Source: CAD feature listing. Evaluate the final solid. Frame: model axes, mm. A direction names the side the tool comes from. Coordinates: 2 decimals unless noted, no trailing zeros. Order: outer loops, then holes, each group sorted by start corner. A loop starts at its lowest first (then second) coordinate and runs counter-clockwise, first axis right, second up. Notation, with made-up numbers: (72, 80.5) -> (111, 80.5) arc R28 cw to (111, 117.5) -> close; hole circle Ø1 at (79.5, 60.25). An arc over 180 degrees is marked (long way). Put each result on its own line as item: value.
from build123d import *

# Parameters (mm, degrees)
SKETCH2_W           = 67
SKETCH2_H           = 85
SKETCH2_W_2         = 57
SKETCH2_H_2         = 75
BOSS_EXTRUDE1_DEPTH = 4
SKETCH2_3_W         = 67
SKETCH2_3_H         = 85
SKETCH2_3_W_2       = 57
SKETCH2_3_H_2       = 75
BOSS_EXTRUDE2_DEPTH = 114
SKETCH4_W           = 67
SKETCH4_H           = 85
SKETCH4_W_2         = 63
SKETCH4_H_2         = 81
BOSS_EXTRUDE3_DEPTH = 25
SKETCH6_R           = 8
CUT_EXTRUDE1_DEPTH  = 25
SKETCH5_W           = 10
SKETCH5_H           = 15
CUT_EXTRUDE2_DEPTH  = 25


with BuildPart() as part:
    # Sketch2 → Boss-Extrude1 (new body)
    # profile 1 of 2: a face of its own
    with BuildSketch(Plane(origin=(0, 0, 0), x_dir=(1, 0, 0), z_dir=(0, 1, 0))):
        Rectangle(SKETCH2_W, SKETCH2_H)
        Rectangle(SKETCH2_W_2, SKETCH2_H_2, mode=Mode.SUBTRACT)
    # profile 2 of 2: a face of its own
    with BuildSketch(Plane(origin=(0, 0, 0), x_dir=(1, 0, 0), z_dir=(0, 1, 0))):
        Rectangle(SKETCH2_W_2, SKETCH2_H_2)
    extrude(amount=BOSS_EXTRUDE1_DEPTH)

    # Sketch2_3 → Boss-Extrude2 (add)
    with BuildSketch(Plane(origin=(0, 0, 0), x_dir=(1, 0, 0), z_dir=(0, 1, 0))):
        Rectangle(SKETCH2_3_W, SKETCH2_3_H)
        Rectangle(SKETCH2_3_W_2, SKETCH2_3_H_2, mode=Mode.SUBTRACT)
    extrude(amount=BOSS_EXTRUDE2_DEPTH)

    # Sketch4 → Boss-Extrude3 (add)
    with BuildSketch(Plane(origin=(0, 114, 0), x_dir=(1, 0, 0), z_dir=(0, 1, 0))):
        Rectangle(SKETCH4_W, SKETCH4_H)
        Rectangle(SKETCH4_W_2, SKETCH4_H_2, mode=Mode.SUBTRACT)
    extrude(amount=BOSS_EXTRUDE3_DEPTH)

    # Sketch6 → Cut-Extrude1 (cut)
    with BuildSketch(Plane.XY.offset(42.5)):
        with Locations((0, 60)):
            Circle(SKETCH6_R)
    extrude(amount=-CUT_EXTRUDE1_DEPTH, mode=Mode.SUBTRACT)

    # Sketch5 → Cut-Extrude2 (cut)
    with BuildSketch(Plane(origin=(0, 0, -42.5), x_dir=(-1, 0, 0), z_dir=(0, 0, -1))):
        with Locations((18.5, 14.5)):
            Rectangle(SKETCH5_W, SKETCH5_H)
    extrude(amount=-CUT_EXTRUDE2_DEPTH, mode=Mode.SUBTRACT)


solid = part.part
1. Pull-direction query (X, two-part tool) for faces 4 (the flat face through (0, 0, -1)), 5 (the flat face through (33.5, 69, 1)), 6 (the flat face through (-13.5, 14, -40)), 7 (the flat face through (-23.5, 14, -40)); classes: pulls with the +X half, pulls with the -X half, needs draft (parallel to the pull), parting line crosses it, or undercut.
Numbers:
face 4: needs draft
face 5: pulls with the +X half
face 6: undercut
face 7: undercut
2. Cut plane A-A on x = 0. Output: boundary loops of the cut face in (y, z), plus the area to 3 significant figures.
Numbers:
outline: (0, -42.5) -> (139, -42.5) -> (139, -40.5) -> (114, -40.5) -> (114, -37.5) -> (4, -37.5) -> (4, 37.5) -> (52, 37.5) -> (52, 42.5) -> (0, 42.5) -> close; (68, 37.5) -> (114, 37.5) -> (114, 40.5) -> (139, 40.5) -> (139, 42.5) -> (68, 42.5) -> close
area: 1,460 mm2
3. First-contact query: pin 1 (6 mm diameter, centred on x = 24.5, z = -21.5, fed in from +Y). Flat tip, straight axial feed; report the tip coordinate or a pass-through.
Numbers:
pin 1: stops at y = 4
4. Set-up query: faces 1 (the flat face through (0, 69, -42.5)), 2 (the flat face through (0, 126, -40.5)), 3 (the flat face through (-18, 22, -40)). Return all of +Z, -Z, +X, -X, +Y, -Y with unobstructed straight access to the full face (end or side cutting, diameter ignored); none if empty.
Numbers:
face 1: -Z, +X, -X, +Y, -Y
face 2: +Y
face 3: -Z
5. Cut plane B-B on y = 60. Output: boundary loops of the cut face in (x, z).
Numbers:
outline: (-33.5, -42.5) -> (33.5, -42.5) -> (33.5, 42.5) -> (8, 42.5) -> (8, 37.5) -> (28.5, 37.5) -> (28.5, -37.5) -> (-28.5, -37.5) -> (-28.5, 37.5) -> (-8, 37.5) -> (-8, 42.5) -> (-33.5, 42.5) -> close
6. Ray query, line 1 along Z through (x, y) = (2, 99); line 2 along X through (y, z) = (23, 12); line 3 along Z through (x, y) = (-28, 131.5). Return the intervals inside material, ascending.
Numbers:
line 1: z = -42.5 to -37.5, 37.5 to 42.5
line 2: x = -33.5 to -28.5, 28.5 to 33.5
line 3: z = -42.5 to -40.5, 40.5 to 42.5
7. Cut plane C-C on z = 4. Output: boundary loops of the cut face in (x, y).
Numbers:
outline: (-33.5, 0) -> (33.5, 0) -> (33.5, 139) -> (31.5, 139) -> (31.5, 114) -> (28.5, 114) -> (28.5, 4) -> (-28.5, 4) -> (-28.5, 114) -> (-31.5, 114) -> (-31.5, 139) -> (-33.5, 139) -> close
8. Cut plane D-D on y = 24. Output: boundary loops of the cut face in (x, z), plus the area to 3 significant figures.
Numbers:
outline: (-33.5, -42.5) -> (33.5, -42.5) -> (33.5, 42.5) -> (-33.5, 42.5) -> close; hole (-28.5, -37.5) -> (28.5, -37.5) -> (28.5, 37.5) -> (-28.5, 37.5) -> close
area: 1,420 mm2
